Autodesk Inventor part; units mm, degrees
ref_plane "YZ Plane" through (0, 0, 0) normal (1, 0, 0) x (0, 1, 0)
ref_plane "XZ Plane" through (0, 0, 0) normal (0, 1, 0) x (-1, 0, 0)
ref_plane "XY Plane" through (0, 0, 0) normal (0, 0, 1) x (1, 0, 0)
sketch "Náčrt1" plane through (0, 0, 0) normal (0, 0, 1) x (1, 0, 0)
  line L0 (-22.5, -10) -> (22.5, -10)
  line L1 (22.5, -10) -> (22.5, 10)
  line L2 (22.5, 10) -> (-22.5, 10)
  line L3 (-22.5, 10) -> (-22.5, -10)
  line L4 (-22.5, -10) -> (22.5, 10) construction
  line L5 (22.5, -10) -> (-22.5, 10) construction
  point P0 (0, 0)
  dimension "d0" = 45
  dimension "d1" = 20
extrude "Vysunutí1" add sketch "Náčrt1" along normal blind 1.5
sketch "Náčrt2" plane through (0, 0, 1.5) normal (0, 0, 1) x (1, 0, 0)
  circle A0 centre (13, 0) radius 8
  circle A1 centre (-13, 0) radius 8
  point P0 (0, 0)
  dimension "d4" = 16
  dimension "d5" = 16
  dimension "d6" = 26
  dimension "d7" = 13
extrude "Vysunutí2" add sketch "Náčrt2" along normal blind 12
sketch "Náčrt3" plane through (0, 0, 1.5) normal (0, 0, 1) x (1, 0, 0)
  line L0 (-4.9518, 7) -> (4.9518, 7) construction
  line L1 (-4.9518, 5.5) -> (4.9518, 5.5)
  line L2 (4.9518, 8.5) -> (-4.9518, 8.5)
  arc A0 (-4.9518, 8.5) -> (-4.9518, 5.5) centre (-4.9518, 7) ccw
  arc A1 (4.9518, 5.5) -> (4.9518, 8.5) centre (4.9518, 7) ccw
  point P0 (0, 0)
  point P1 (0, 7)
  dimension "d10" = 3
  dimension "d11" = 7
extrude "Vysunutí3" add sketch "Náčrt3" along normal blind 2
fillet "Zaoblení1" radius 1 4 edges at (0, 8.5, 3.5) (-6.4518, 7, 3.5) (0, 5.5, 3.5) (6.4518, 7, 3.5)
sketch "Náčrt4" plane through (0, 0, 1.5) normal (0, 0, 1) x (1, 0, 0)
  circle A0 centre (21, 8.75) radius 1
  circle A1 centre (-21, -8.75) radius 1
  point P0 (0, 0)
  dimension "d15" = 2
  dimension "d16" = 2
  dimension "d17" = 17.5
  dimension "d18" = 42
  dimension "d19" = 8.75
  dimension "d20" = 21
extrude "Vysunutí4" cut sketch "Náčrt4" against normal through all
sketch "Náčrt6" plane through (0, 0, 0) normal (1, 0, 0) x (0, 1, 0)
  line L0 (-10, 0) -> (10, 0)
  line L1 (-10, 0) -> (-8, 0)
  line L2 (-8, 0) -> (-8, -2)
  line L3 (-8, -2) -> (-10, -2)
  line L4 (-10, -2) -> (-10, 0)
  line L5 (-8, -2) -> (-16, -2)
  line L6 (-16, -2) -> (-16, -3)
  line L7 (-16, -3) -> (-8, -3)
  line L8 (-8, -3) -> (-8, -2)
  point P0 (0, 0)
  dimension "d23" = 2
  dimension "d24" = 2
  dimension "d25" = 8
  dimension "d26" = 1
extrude "Vysunutí5" add sketch "Náčrt6" along normal mid plane 13
properties part number "UltraZvuk"
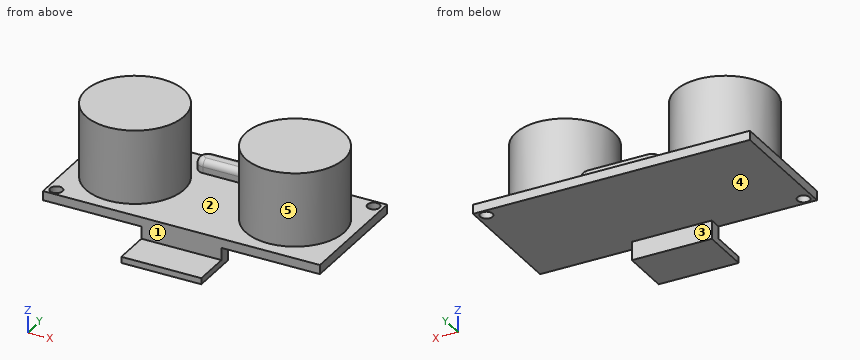
Work out the finished part from the listing and answer in its coordinate system (mm). Face numbers are marked on the shaded views. A direction names the side the tool comes from. Round coordinates to 2 decimals unless told otherwise and drop trailing zeros. Loops run counter-clockwise (first coordinate to the right, second up) from the corner with the lowest first, then second, coordinate; pieces in that order, holes last.
(1) Find the intervals of material crossed by L1, parallel to Y at x = 21, z = 0.8; L2, parallel to Y at x = -21, z = 1.1; L3, parallel to Y at x = -3.5, z = 2, in increasing order.
Computed values:
L1: y = -10 to 7.75, 9.75 to 10
L2: y = -10 to -9.75, -7.75 to 10
L3: y = 5.5 to 8.5
(2) The mould has two halves that part along X. Classify the marked faces 4 and 5: pulls with the +X half, pulls with the -X half, needs draft (parallel to the pull), parting line crosses it, or undercut.
Computed values:
face 4: needs draft
face 5: undercut
(3) For the marked faces 1, 2 and 3, determine the directions among +Z, -Z, +X, -X, +Y, -Y from which every point of the face is accessible in a straight line to the end or side of a thin tool.
Computed values:
face 1: +Z, +X, -X, -Y
face 2: +Z
face 3: -Z, +X, -X, +Y
(4) The part is cut by section A-A, the plane y = -8.75. Give the vertices of the cut face in (x, z), and give its area (4 significant figures).
Computed values:
outline: (-22.5, 0) - (-22, 0) - (-22, 1.5) - (-22.5, 1.5) - close; (-20, 0) - (-6.5, 0) - (-6.5, -3) - (6.5, -3) - (6.5, 0) - (22.5, 0) - (22.5, 1.5) - (-20, 1.5) - close
area: 103.5 mm2
(5) The part is cut by section B-B, the plane x = 13. Give the vertices of the cut face in (y, z).
Computed values:
outline: (-10, 0) - (10, 0) - (10, 1.5) - (8, 1.5) - (8, 13.5) - (-8, 13.5) - (-8, 1.5) - (-10, 1.5) - close
(6) The part is cut by section D-D, the plane z = 5.5. Give the vertices of the cut face in (x, y).
Computed values:
outline: circle Ø16 at (-13, 0); circle Ø16 at (13, 0)
(7) Each of these flat-tipped pins is pushed along its axis until it touches: P1, Ø0.9, axis at x = 1, z = -1.5, coming from the +Y side; P2, Ø1.8, axis at x = -0.5, z = 0, coming from the -Y side; P3, Ø1, axis at x = -8.5, y = -7.5, coming from the -Z side. Where does it stop, or does it pass through?
Computed values:
P1: stops at y = -8
P2: stops at y = -10
P3: stops at z = 0
(8) The part is cut by section C-C, the plane y = 0. Give the vertices of the cut face in (x, z).
Computed values:
outline: (-22.5, 0) - (22.5, 0) - (22.5, 1.5) - (21, 1.5) - (21, 13.5) - (5, 13.5) - (5, 1.5) - (-5, 1.5) - (-5, 13.5) - (-21, 13.5) - (-21, 1.5) - (-22.5, 1.5) - close
